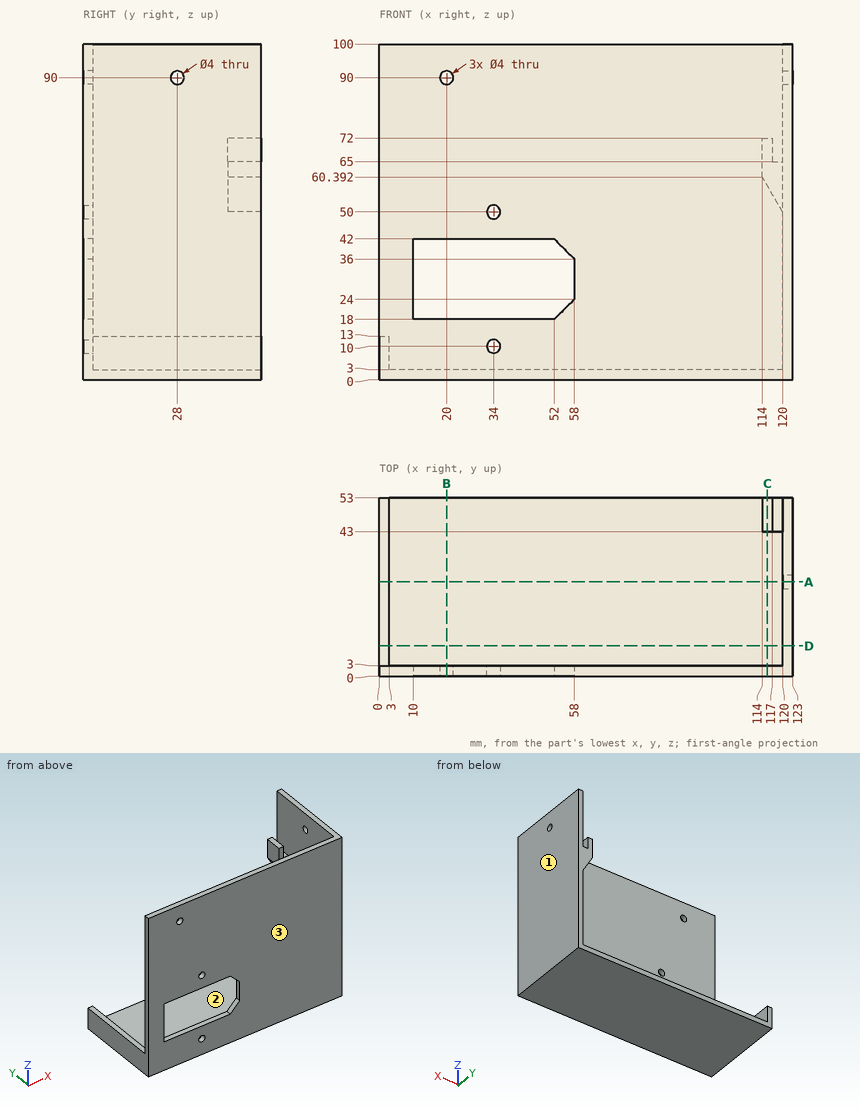
Here's the drawing with two shaded views (mm, measured from the low corner). I have some questions. Give positions to 0.01 mm unless a question says otherwise; leave off trailing zeros. Loops run counter-clockwise (first coordinate to the right, second up) from the corner with the lowest first, then second, coordinate; pieces in that order, holes last. Notation, with made-up numbers: M -21,79.5 L -7,79.5 A13 cw -7,91.5 Z; hole C -34.75,-18 d10. An arc over 180 degrees is marked long. Answer in a Markdown table with one row per item.
1. If I drill on line 1 along Z through (x, y) = (34, 0.75); line 2 along X through (y, z) = (7.5, 5.5); line 3 along Z through (x, y) = (20, 1.35), over which ranges is the centre line in solid material (lowest first)?
Taken from the geometry:
| item | result |
|---|---|
| line 1 | z = 0 to 8, 12 to 18, 42 to 48, 52 to 100 |
| line 2 | x = 0 to 3, 120 to 123 |
| line 3 | z = 0 to 18, 42 to 88, 92 to 100 |
2. Suppose I cut it at C-C on x = 115.5. Write out the boundary of the cut face in (y, z).
Taken from the geometry:
| item | result |
|---|---|
| outline | M 0,0 L 53,0 L 53,3 L 3,3 L 3,100 L 0,100 Z; M 43,57.79 L 53,57.79 L 53,72 L 43,72 Z |
3. Suppose I cut it at D-D on y = 9. Write out the boundary of the cut face in (x, z).
Taken from the geometry:
| item | result |
|---|---|
| outline | M 0,0 L 123,0 L 123,100 L 120,100 L 120,3 L 3,3 L 3,13 L 0,13 Z |
4. Suppose I cut it at A-A on y = 28. Write out the boundary of the cut face in (x, z), plus the area to 3 significant figures.
Taken from the geometry:
| item | result |
|---|---|
| outline | M 0,0 L 123,0 L 123,88 L 120,88 L 120,3 L 3,3 L 3,13 L 0,13 Z; M 120,92 L 123,92 L 123,100 L 120,100 Z |
| area | 678 mm² |
5. Suppose I cut it at B-B on x = 20. Write out the boundary of the cut face in (y, z).
Taken from the geometry:
| item | result |
|---|---|
| outline | M 0,0 L 53,0 L 53,3 L 3,3 L 3,18 L 0,18 Z; M 0,42 L 3,42 L 3,88 L 0,88 Z; M 0,92 L 3,92 L 3,100 L 0,100 Z |
6. Thinking about a two-plate mould opening in X: for the marked faces 1, 2 and 3, which applies, released by +X, released by -X, zero draft, split by the parting line, or undercut?
Taken from the geometry:
| item | result |
|---|---|
| face 1 | released by +X |
| face 2 | undercut |
| face 3 | zero draft |
7. For pin 1 Ø4.5 at (y, z) = (28, 90) entering from -X; pin 2 Ø1.5 at (x, y) = (17, 23) entering from +Z; pin 3 Ø0.9 at (x, y) = (118, 48) entering from +Z, each with a flat end and sliding along its axis, tell me the tip position at first contact or that it passes through.
Taken from the geometry:
| item | result |
|---|---|
| pin 1 | stops at x = 120 |
| pin 2 | stops at z = 3 |
| pin 3 | stops at z = 65 |
